Geometry: final body of the model. Coordinates: model frame, mm. A direction names the side the tool comes from. Coordinates: 2 decimals unless noted, no trailing zeros. Order: outer loops, then holes, each group sorted by start corner. A loop starts at its lowest first (then second) coordinate and runs counter-clockwise, first axis right, second up. Notation, with made-up numbers: (-31, 75.5) - (8, 75.5) arc R23 cw to (8, 109.5) - close; hole circle Ø4 at (-18, 80). An arc over 180 degrees is marked (long way). Use a Markdown table: item, result. Add a question column.
Autodesk Inventor part; units mm, degrees
ref_plane "YZ Plane" through (0, 0, 0) normal (1, 0, 0) x (0, 1, 0)
ref_plane "XZ Plane" through (0, 0, 0) normal (0, 1, 0) x (-1, 0, 0)
ref_plane "XY Plane" through (0, 0, 0) normal (0, 0, 1) x (1, 0, 0)
sketch "Sketch1" plane through (0, 0, 0) normal (0, 1, 0) x (-1, 0, 0)
  line L0 (-12.7, -12.7) -> (12.7, -12.7)
  line L1 (12.7, -12.7) -> (12.7, 12.7)
  line L2 (12.7, 12.7) -> (-12.7, 12.7)
  line L3 (-12.7, 12.7) -> (-12.7, -12.7)
  line L4 (-12.7, -12.7) -> (12.7, 12.7) construction
  line L5 (12.7, -12.7) -> (-12.7, 12.7) construction
  line L6 (9.525, 9.525) -> (9.525, -9.525)
  line L7 (9.525, -9.525) -> (-9.525, -9.525)
  line L8 (-9.525, -9.525) -> (-9.525, 9.525)
  line L9 (-9.525, 9.525) -> (9.525, 9.525)
  point P0 (0, 0)
  dimension "d0" = 25.4
  dimension "d1" = 25.4
  dimension "d2" = 3.175
extrude "Extrusion1" add sketch "Sketch1" along normal blind 201.5942
sketch "Sketch2" plane through (12.7, 0, 12.7) normal (1, 0, 0) x (0, 0, -1)
  line L0 (0, 0) -> (25.4, 0)
  line L1 (25.4, 0) -> (25.4, 201.5942)
  line L2 (0, 201.5942) -> (25.4, 201.5942)
  line L3 (0, 0) -> (0, 201.5942)
  line L4 (0, 201.5942) -> (25.4, 188.4235)
  point P0 (12.7, 0)
  dimension "d5" = 27.408
extrude "Extrusion2" [suppressed]
sketch "Sketch3" plane through (12.7, 0, 12.7) normal (1, 0, 0) x (0, 0, -1)
  line L0 (0, 201.5942) -> (0, 215.9)
  line L1 (25.4, 201.5942) -> (25.4, 215.9)
  line L2 (25.4, 215.9) -> (0, 215.9)
  line L3 (25.4, 241.3) -> (0, 241.3) construction
  line L4 (0, 241.3) -> (0, 215.9) construction
  line L5 (0, 215.9) -> (25.4, 215.9) construction
  line L6 (25.4, 215.9) -> (25.4, 241.3) construction
  line L7 (25.4, 241.3) -> (0, 215.9) construction
  line L8 (0, 241.3) -> (25.4, 215.9) construction
  circle A0 centre (12.7, 206.375) radius 3.2512
  circle A1 centre (12.7, 228.6) radius 2.4892 construction
  circle A2 centre (12.7, 184.15) radius 3.2512
  line L9 (0, 201.5942) -> (25.4, 201.5942)
  point P0 (12.7, 0)
  dimension "d8" = 14.3058
  dimension "d9" = 25.4
  dimension "d10" = 25.4
  dimension "d11" = 6.5024
  dimension "d12" = 4.9784
  dimension "d13" = 22.225
  dimension "d14" = 22.225
extrude "Extrusion3" cut sketch "Sketch3" against normal through all contours A2
sketch "Sketch4" plane through (12.7, 0, -12.7) normal (0, 0, -1) x (-1, 0, 0)
  circle A0 centre (12.7, 25.4) radius 3.2512
  circle A1 centre (12.7, 50.8) radius 3.2512
  line L0 (0, 0) -> (25.4, 0)
  point P0 (12.7, 0)
  point P1 (12.7, 0)
  point P2 (12.7, 0)
  dimension "d17" = 6.5024
  dimension "d18" = 6.5024
  dimension "d19" = 25.4
  dimension "d20" = 25.4
extrude "Extrusion4" cut sketch "Sketch4" against normal blind 25.4
sketch "Sketch5" plane through (-12.7, 0, 12.7) normal (0, 0, 1) x (1, 0, 0)
  circle A0 centre (12.7, 25.4) radius 3.2512 construction
  circle A1 centre (12.7, 50.8) radius 3.2512 construction
  line L0 (15.9512, 25.4) -> (15.9512, 50.8) construction
  line L1 (9.4488, 25.4) -> (9.4488, 50.8) construction
  arc A2 (9.4488, 25.4) -> (15.9512, 25.4) centre (12.7, 25.4) ccw construction
  arc A3 (15.9512, 50.8) -> (9.4488, 50.8) centre (12.7, 50.8) ccw construction
  line L2 (18.4912, 50.8) -> (18.4912, 25.4)
  arc A4 (6.9088, 25.4) -> (18.4912, 25.4) centre (12.7, 25.4) ccw
  line L3 (6.9088, 25.4) -> (6.9088, 50.8)
  arc A5 (18.4912, 50.8) -> (6.9088, 50.8) centre (12.7, 50.8) ccw
  point P0 (12.7, 0)
  dimension "d26" = 2.54
extrude "Extrusion5" cut sketch "Sketch5" against normal blind 3.175
sketch "Sketch6" plane through (12.7, 0, 12.7) normal (1, 0, 0) x (0, 0, -1)
  line L0 (12.7, 0) -> (12.7, 6.5024)
  circle A0 centre (12.7, -12.7) radius 3.2512
  line L1 (0, 0) -> (25.4, 0)
  circle A1 centre (12.7, 12.7) radius 3.2512
  circle A2 centre (12.7, 38.1) radius 3.2512
  circle A3 centre (12.7, 63.5) radius 3.2512
  line L2 (12.7, -12.7) -> (12.7, 63.5) construction
  dimension "d27" = 6.5024
  dimension "d31" = 25.4
  dimension "d38" = 6.5024
  dimension "d39" = 12.7
extrude "Extrusion6" cut sketch "Sketch6" against normal blind 25.4 contours A1 | A2 | A3
extrude "Extrusion7" add sketch "Sketch3" against normal blind 25.4 contours L0 L2 L1 L9
sketch "Sketch7" plane through (12.7, 215.9, 12.7) normal (0, 1, 0) x (1, 0, 0)
  line L0 (0, 25.4) -> (0, 0)
  line L1 (0, 25.4) -> (-25.4, 25.4)
  line L2 (-25.4, 0) -> (-25.4, 25.4)
  line L3 (0, 0) -> (-25.4, 0)
  line L4 (-22.225, 22.225) -> (-3.175, 22.225)
  line L5 (-3.175, 22.225) -> (-3.175, 3.175)
  line L6 (-3.175, 3.175) -> (-22.225, 3.175)
  line L7 (-22.225, 3.175) -> (-22.225, 22.225)
  point P0 (-12.7, 12.7)
  dimension "d42" = 3.175
extrude "Extrusion8" cut sketch "Sketch7" against normal blind 25.4 contours L4 L5 L6 L7
properties part number "STRU_014_BilletPole_9in_Angled" material "Aluminum 6061"
1) Section query A-A (y = 12.7). Return the cut outline in (x, z) (3 decimals).
2) Section query C-C (z = -7.25). Return the cut outline in (x, y) (3 decimals), and give its area (3 significant figures).
3) Section query B-B (x = 0). Return the cut outline in (y, z) (3 decimals).
4) Line query: line 1 (Y direction, x = 10.95, z = 0); line 2 (X direction, y = 202, z = 3.5) (3 decimals). Output: solid intervals per line, ascending. Write a range as from..to.
5) Draft query along Y for faces 3 (the flat face through (0, 215.9, 11)), 4 (the cylindrical face through (0.705, 47.626, -11.135)), 5 (the cylindrical face through (0.13, 56.59, 11.13)), 6 (the flat face through (-12.7, 109, 0)). Return one class per face: released by +Y, released by -Y, zero draft, split by the parting line, or undercut.
6) Section query D-D (y = 38.1). Return the cut outline in (x, z) (3 decimals).
7) First-contact query: pin 1 (10.5 mm diameter, centred on x = 0, y = 50.8, fed in from +Z) (3 decimals). Flat tip, straight axial feed; report the tip coordinate or a pass-through.
8) Access query for faces 1 (the flat face through (0, 109, 9.525)), 2 (the flat face through (-11, 0, 0)). Directions: +Z, -Z, +X, -X, +Y, -Y. A direction counts if a zero-diameter tool reaches every point of the face in a straight line with its end or side. Return the directions, or none.
From the geometry:
| question | item | result |
|---|---|---|
| 1 | outline | (-12.7, -12.7) - (12.7, -12.7) - (12.7, -3.251) - (9.525, -3.251) - (9.525, -9.525) - (-9.525, -9.525) - (-9.525, -3.251) - (-12.7, -3.251) - close; (-12.7, 3.251) - (-9.525, 3.251) - (-9.525, 9.525) - (9.525, 9.525) - (9.525, 3.251) - (12.7, 3.251) - (12.7, 12.7) - (-12.7, 12.7) - close |
| 2 | outline | (-12.7, 0) - (-9.525, 0) - (-9.525, 215.9) - (-12.7, 215.9) - close; (9.525, 0) - (12.7, 0) - (12.7, 215.9) - (9.525, 215.9) - close |
| 2 | area | 1,370 mm^2 |
| 3 | outline | (0, -12.7) - (22.149, -12.7) - (22.149, -9.525) - (0, -9.525) - close; (0, 9.525) - (19.609, 9.525) - (19.609, 12.7) - (0, 12.7) - close; (28.651, -12.7) - (47.549, -12.7) - (47.549, -9.525) - (28.651, -9.525) - close; (54.051, -12.7) - (215.9, -12.7) - (215.9, -9.525) - (54.051, -9.525) - close; (56.591, 9.525) - (215.9, 9.525) - (215.9, 12.7) - (56.591, 12.7) - close |
| 4 | line 1 | y = 0..9.45, 15.95..34.85, 41.35..60.25, 66.75..180.9, 187.4..203.12, 209.63..215.9 |
| 4 | line 2 | x = -12.7..-9.525, 9.525..12.7 |
| 5 | face 3 | released by +Y |
| 5 | face 4 | undercut |
| 5 | face 5 | undercut |
| 5 | face 6 | zero draft |
| 6 | outline | (-12.7, -12.7) - (12.7, -12.7) - (12.7, -3.251) - (9.525, -3.251) - (9.525, -9.525) - (-9.525, -9.525) - (-9.525, -3.251) - (-12.7, -3.251) - close; (-12.7, 3.251) - (-9.525, 3.251) - (-9.525, 9.525) - (-5.791, 9.525) - (-5.791, 12.7) - (-12.7, 12.7) - close; (5.791, 9.525) - (9.525, 9.525) - (9.525, 3.251) - (12.7, 3.251) - (12.7, 12.7) - (5.791, 12.7) - close |
| 7 | pin 1 | stops at z = -9.525 |
| 8 | face 1 | +Y, -Y |
| 8 | face 2 | +Z, -Z, +X, -X, -Y |
